Design review of the part built by this model. Coordinates are the model's own, in mm. A direction names the side the tool comes from. Coordinates: 2 decimals unless noted, no trailing zeros. Loops run counter-clockwise (first coordinate to the right, second up) from the corner with the lowest first, then second, coordinate; pieces in that order, holes last.
Q1. Add section B-B on x = -1. Give the boundary of the cut face in (y, z) (3 decimals).
Q2. Machinability: for faces 1 (the face through (-21.068, 87.198, 28.209)), 2 (the face through (59.69, 48, 0)), 3 (the face through (48.26, 100, -12)), 4 (the face through (59.69, 100, 0)), which of the approach directions +Z, -Z, +X, -X, +Y, -Y give a long, thin tool a straight path to every point of the face, cutting with its end or side? Answer none if there is none.
Q3. Draft analysis for pull direction Z (two halves, no side actions). For faces 5 (the face through (22.86, 104, 0)), 6 (the face through (29, 104, 6.35)), 7 (the face through (48.26, 100, 12)), 8 (the face through (28.513, 104.823, -0.716)), state which applies: released by +Z, released by -Z, zero draft, split by the parting line, or undercut.
Q4. Add section C-C on y = 64. Give the boundary of the cut face in (x, z).
Q5. Add section A-A on z = -15.5. Give the boundary of the cut face in (x, y).
Q6. For P1, Ø23, axis at x = 7, z = -15, coming from the +Y side; P2, Ø5.5, axis at x = 31, y = 105, coming from the +Z side; P3, Ø5.5, axis at y = 103, z = -2, coming from the -X side; P4, Ø6, axis at x = 22, z = 27, coming from the -Y side, all flat-tipped, find the tip position at first contact; note any pin that passes through.
Q7. Add section D-D on x = 54. Give the boundary of the cut face in (y, z).
Q8. Wall thickness on probe 1 along X at (y, z) = (91, -10); probe 2 along X at (y, z) = (88.9, 29); probe 3 along X at (y, z) = (34.5, -5.5): over which ranges is each line inside the solid? List them lowest first.
```python
from build123d import *

# Parameters (mm, degrees)
SKETCH1_W                           = 127
SKETCH1_H                           = 76.2
MAIN_BODY_DEPTH                     = 101.6
HOLLOW_IT_T                         = -3.81
HOLE_FOR_SCROLLWHEEL_REACH          = 127.724
SKETCH2_W                           = 12.7
SKETCH2_H                           = 40.64
NIBBLE_BASE_HOLE_DEPTH              = 12.7
NIBBLE_HOLE_DEPTH                   = 24.13
NIBBLE_HOLE_DEPTH_BACK              = 11.43
SKETCH5_R                           = 3.302
EASY_TO_INSERT_SCROLL_WHEEL_R       = 2.54
SKETCH6_W                           = 57.15
SKETCH6_H                           = 44.45
HOLE_FOR_JOYSTICK_DEPTH             = 11.43
SKETCH10_W                          = 44.45
SKETCH10_H                          = 6.985
SKETCH10_W_2                        = 31.75
BOX_NIBBLE_BASE_DEPTH               = 15.24
SKETCH11_W                          = 4.572
SKETCH11_H                          = 24.856466434
SKETCH11_W_2                        = 2.948658359
ARCH_NIBBLE_BASE_DEPTH              = 17.78
ARCH_NIBBLE_HOLES_REACH             = 134.21
SKETCH12_R                          = 3.81
ARCH_NIBBLE_HOLES_DIRECTION_2_REACH = 134.21
BOX_NIBBLE_HOLES_REACH              = 141.158
SKETCH13_R                          = 4.445
BOX_NIBBLE_HOLES_DIRECTION_2_REACH  = 141.158


with BuildPart() as part:
    # Sketch1 → main body (new body)
    with BuildSketch(Plane(origin=(0, 0, 0), x_dir=(1, 0, 0), z_dir=(0, 1, 0))):
        Rectangle(SKETCH1_W, SKETCH1_H)
    extrude(amount=MAIN_BODY_DEPTH)

    # hollow it
    hollow_it_openings = [part.faces().sort_by_distance(p)[0] for p in [
        (0, 0, 0),
    ]]
    offset(amount=HOLLOW_IT_T, openings=hollow_it_openings, kind=Kind.INTERSECTION)

    # Sketch2 → hole for scrollwheel (cut, up to next)
    with BuildSketch(Plane(origin=(0, 101.6, 0), x_dir=(1, 0, 0), z_dir=(0, 1, 0)), mode=Mode.PRIVATE) as hole_for_scrollwheel_sk1:
        with Locations((41.91, 0)):
            Rectangle(SKETCH2_W, SKETCH2_H)
    hole_for_scrollwheel_tool1 = extrude(hole_for_scrollwheel_sk1.sketch, amount=-HOLE_FOR_SCROLLWHEEL_REACH, mode=Mode.PRIVATE) & part.part
    add(hole_for_scrollwheel_tool1.solids().sort_by_distance((41.91, 101.6, 0))[0], mode=Mode.SUBTRACT)

    # Sketch3 → nibble base hole (add)
    with BuildSketch(Plane(origin=(35.56, 0, 0), x_dir=(0, 0, -1), z_dir=(1, 0, 0))):
        Polygon((0, 101.6), (6.35, 101.6), (6.35, 106.68), (-6.35, 106.68), (-6.35, 101.6), align=None)
    extrude(amount=-NIBBLE_BASE_HOLE_DEPTH)

    # Sketch5 → nibble hole (cut, two sides: drawn at the far end of the back side and taken through both)
    with BuildSketch(Plane(origin=(35.56, 0, 0), x_dir=(0, 0, -1), z_dir=(1, 0, 0)).offset(-NIBBLE_HOLE_DEPTH_BACK)):
        with Locations(Location((0, 101.6, 0), (0, 0, 180))):
            Circle(SKETCH5_R)
    extrude(amount=NIBBLE_HOLE_DEPTH + NIBBLE_HOLE_DEPTH_BACK, mode=Mode.SUBTRACT)

    # easy to insert scroll wheel
    # the kernel refuses this fillet: 2.54 mm, written as the material it takes off along each edge
    with BuildSketch(Plane(origin=(48.26, 101.6, 0), x_dir=(0, 0.9999950652018582, -0.0031415874858792044), z_dir=(0, 0.0031415874858792044, 0.9999950652018582))) as easy_to_insert_scroll_wheel_piece_1:
        with BuildLine():
            CenterArc((3.302 + EASY_TO_INSERT_SCROLL_WHEEL_R, -EASY_TO_INSERT_SCROLL_WHEEL_R), EASY_TO_INSERT_SCROLL_WHEEL_R, 90, 90)
            Line((3.302, -EASY_TO_INSERT_SCROLL_WHEEL_R), (3.302, 0))
            Line((3.302, 0), (3.302 + EASY_TO_INSERT_SCROLL_WHEEL_R, 0))
        make_face()
    revolve(axis=Axis((48.26, 101.6, 0), (-1, 0, 0)), revolution_arc=359.64, mode=Mode.SUBTRACT)
    with BuildSketch(Plane(origin=(35.56, 101.6, 0), x_dir=(0, 0, 1), z_dir=(0, 1, 0))) as easy_to_insert_scroll_wheel_piece_2:
        with BuildLine():
            CenterArc((3.302 + EASY_TO_INSERT_SCROLL_WHEEL_R, -EASY_TO_INSERT_SCROLL_WHEEL_R), EASY_TO_INSERT_SCROLL_WHEEL_R, 90, 90)
            Line((3.302, -EASY_TO_INSERT_SCROLL_WHEEL_R), (3.302, 0))
            Line((3.302, 0), (3.302 + EASY_TO_INSERT_SCROLL_WHEEL_R, 0))
        make_face()
    revolve(axis=Axis((35.56, 101.6, 0), (1, 0, 0)), mode=Mode.SUBTRACT)

    # Sketch6 → hole for joystick (cut)
    with BuildSketch(Plane(origin=(0, 101.6, 0), x_dir=(1, 0, 0), z_dir=(0, 1, 0))):
        with Locations((-25.173658359, 0)):
            Rectangle(SKETCH6_W, SKETCH6_H)
    extrude(amount=-HOLE_FOR_JOYSTICK_DEPTH, mode=Mode.SUBTRACT)

    # Sketch10 → box nibble base (add)
    with BuildSketch(Plane.XZ.offset(-97.79)):
        with Locations((-25.173658359, 28.2575)):
            Rectangle(SKETCH10_W, SKETCH10_H)
        with Locations((-25.173658359, -28.2575)):
            Rectangle(SKETCH10_W_2, SKETCH10_H)
    extrude(amount=BOX_NIBBLE_BASE_DEPTH)

    # Sketch11 → arch nibble base (add)
    with BuildSketch(Plane.XZ.offset(-97.79)):
        with Locations((6.957341641, 0)):
            Rectangle(SKETCH11_W, SKETCH11_H)
        with Locations((-57.354329179, 0)):
            Rectangle(SKETCH11_W_2, SKETCH11_H)
    extrude(amount=ARCH_NIBBLE_BASE_DEPTH)

    # arch nibble holes: up to this face of the body (flat: up to its plane)
    arch_nibble_holes_end = Plane(part.part.faces().sort_by_distance((9.243341641, 88.9, 0))[0])
    # Sketch12 → arch nibble holes (cut, up to the picked face)
    with BuildSketch(Plane.ZY.offset(-4.671341641), mode=Mode.PRIVATE) as arch_nibble_holes_sk1:
        with Locations((0, 91.44)):
            Circle(SKETCH12_R)
    arch_nibble_holes_tool1 = split(extrude(arch_nibble_holes_sk1.sketch, amount=-ARCH_NIBBLE_HOLES_REACH, mode=Mode.PRIVATE), bisect_by=arch_nibble_holes_end, keep=Keep.BOTH, mode=Mode.PRIVATE)
    add(arch_nibble_holes_tool1.solids().sort_by(Axis((4.671342, 91.44, 0), (1, 0, 0)))[0], mode=Mode.SUBTRACT)

    # arch nibble holes direction 2: up to this face of the body (flat: up to its plane)
    arch_nibble_holes_direction_2_end = Plane(part.part.faces().sort_by_distance((-59.69, 48.895, 0))[0])
    # Sketch12 → arch nibble holes direction 2 (cut, up to the picked face)
    with BuildSketch(Plane.ZY.offset(-4.671341641), mode=Mode.PRIVATE) as arch_nibble_holes_direction_2_sk1:
        with Locations((0, 91.44)):
            Circle(SKETCH12_R)
    arch_nibble_holes_direction_2_tool1 = split(extrude(arch_nibble_holes_direction_2_sk1.sketch, amount=ARCH_NIBBLE_HOLES_DIRECTION_2_REACH, mode=Mode.PRIVATE), bisect_by=arch_nibble_holes_direction_2_end, keep=Keep.BOTH, mode=Mode.PRIVATE)
    add(arch_nibble_holes_direction_2_tool1.solids().sort_by(Axis((4.671342, 91.44, 0), (-1, 0, 0)))[0], mode=Mode.SUBTRACT)

    # box nibble holes: up to this face of the body (flat: up to its plane)
    box_nibble_holes_end = Plane(part.part.faces().sort_by_distance((0, 48.895, -34.29))[0])
    # Sketch13 → box nibble holes (cut, up to the picked face)
    with BuildSketch(Plane.XY.offset(-24.765), mode=Mode.PRIVATE) as box_nibble_holes_sk1:
        with Locations((-25.173658359, 88.9)):
            Circle(SKETCH13_R)
    box_nibble_holes_tool1 = split(extrude(box_nibble_holes_sk1.sketch, amount=-BOX_NIBBLE_HOLES_REACH, mode=Mode.PRIVATE), bisect_by=box_nibble_holes_end, keep=Keep.BOTH, mode=Mode.PRIVATE)
    add(box_nibble_holes_tool1.solids().sort_by(Axis((-25.173658, 88.9, -24.765), (0, 0, -1)))[0], mode=Mode.SUBTRACT)

    # box nibble holes direction 2: up to this face of the body (flat: up to its plane)
    box_nibble_holes_direction_2_end = Plane(part.part.faces().sort_by_distance((0, 48.895, 34.29))[0])
    # Sketch13 → box nibble holes direction 2 (cut, up to the picked face)
    with BuildSketch(Plane.XY.offset(-24.765), mode=Mode.PRIVATE) as box_nibble_holes_direction_2_sk1:
        with Locations((-25.173658359, 88.9)):
            Circle(SKETCH13_R)
    box_nibble_holes_direction_2_tool1 = split(extrude(box_nibble_holes_direction_2_sk1.sketch, amount=BOX_NIBBLE_HOLES_DIRECTION_2_REACH, mode=Mode.PRIVATE), bisect_by=box_nibble_holes_direction_2_end, keep=Keep.BOTH, mode=Mode.PRIVATE)
    add(box_nibble_holes_direction_2_tool1.solids().sort_by(Axis((-25.173658, 88.9, -24.765), (0, 0, 1)))[0], mode=Mode.SUBTRACT)


solid = part.part
```
Entries:
1. outline: (0, -38.1) - (101.6, -38.1) - (101.6, -22.225) - (97.79, -22.225) - (97.79, -34.29) - (0, -34.29) - close; (0, 34.29) - (97.79, 34.29) - (97.79, 22.225) - (101.6, 22.225) - (101.6, 38.1) - (0, 38.1) - close
2. face 1: none
2. face 2: -Y
2. face 3: +Y, -Y
2. face 4: +Y
3. face 5: zero draft
3. face 6: released by +Z
3. face 7: undercut
3. face 8: undercut
4. outline: (-63.5, -38.1) - (63.5, -38.1) - (63.5, 38.1) - (-63.5, 38.1) - close; hole (-59.69, -34.29) - (59.69, -34.29) - (59.69, 34.29) - (-59.69, 34.29) - close
5. outline: (-63.5, 0) - (-59.69, 0) - (-59.69, 97.79) - (-53.75, 97.79) - (-53.75, 101.6) - (-63.5, 101.6) - close; (3.4, 97.79) - (35.56, 97.79) - (35.56, 101.6) - (3.4, 101.6) - close; (48.26, 97.79) - (59.69, 97.79) - (59.69, 0) - (63.5, 0) - (63.5, 101.6) - (48.26, 101.6) - close
6. P1: stops at y = 101.6
6. P2: stops at z = 6.35
6. P3: stops at x = -63.5
6. P4: stops at y = 97.79
7. outline: (0, -38.1) - (101.6, -38.1) - (101.6, -3.3) arc R3.3 cw to (101.6, 3.3) - (101.6, 38.1) - (0, 38.1) - (0, 34.29) - (97.79, 34.29) - (97.79, -34.29) - (0, -34.29) - close
8. probe 1: x = -63.5 to -59.69, -58.83 to -55.88, 4.67 to 9.24, 59.69 to 63.5
8. probe 2: x = -63.5 to -59.69, -47.4 to -29.62, -20.73 to -2.95, 59.69 to 63.5
8. probe 3: x = -63.5 to -59.69, 59.69 to 63.5
